from build123d import *

# Parameters (mm, degrees)
SKICA1_R                 = 26
P_IDAT_VYSUNUT_M1_DEPTH  = 90
ZAOBLIT1_R               = 2
SKICA2_R                 = 13
P_IDAT_VYSUNUT_M2_DEPTH  = 6.5
SKICA4_R                 = 1.6
ODEBRAT_VYSUNUT_M1_DEPTH = 10
P_IDAT_START             = 6.5
SKICA5_R                 = 13
P_IDAT_VYSUNUT_M4_DEPTH  = 6.5
ZKOSEN_1_SIZE            = 0.5
SKICA8_R                 = 4
ODEBRAT_VYSUNUT_M3_DEPTH = 110.366356825


with BuildPart() as part:
    # Skica1 → Přidat vysunutím1 (new body)
    with BuildSketch(Plane.XY):
        with Locations(Location((0, 0, 0), (0, 0, 180))):
            Circle(SKICA1_R)
    extrude(amount=P_IDAT_VYSUNUT_M1_DEPTH)

    # Zaoblit1
    zaoblit1_edges = [part.edges().sort_by_distance(p)[0] for p in [
        (26, 0, 0),
        (26, 0, 90),
    ]]
    fillet(zaoblit1_edges, radius=ZAOBLIT1_R)

    # Skica2 → Přidat vysunutím2 (add)
    with BuildSketch(Plane(origin=(0, 0, 0), x_dir=(-1, 0, 0), z_dir=(0, 0, -1))):
        with Locations(Location((0, 0, 0), (0, 0, 180))):
            Circle(SKICA2_R)
    extrude(amount=P_IDAT_VYSUNUT_M2_DEPTH)

    # Skica4 → Odebrat vysunutím1 (cut)
    with BuildSketch(Plane(origin=(0, 0, 0), x_dir=(-1, 0, 0), z_dir=(0, 0, -1))):
        with Locations((-17.5, 0)):
            Circle(SKICA4_R)
        with Locations((0, 17.5)):
            Circle(SKICA4_R)
        with Locations((17.5, 0)):
            Circle(SKICA4_R)
        with Locations((0, -17.5)):
            Circle(SKICA4_R)
    extrude(amount=-ODEBRAT_VYSUNUT_M1_DEPTH, mode=Mode.SUBTRACT)

    # Skica5 → Přidat vysunutím4 (add)
    with BuildSketch(Plane.XY.offset(90).offset(P_IDAT_START)):
        Circle(SKICA5_R)
    extrude(amount=-P_IDAT_VYSUNUT_M4_DEPTH)

    # Zkosení1
    zkosen_1_edges = [part.edges().sort_by_distance(p)[0] for p in [
        (-13, 0, -6.5),
        (-13, 0, 96.5),
    ]]
    chamfer(zkosen_1_edges, length=ZKOSEN_1_SIZE)

    # Skica8 → Odebrat vysunutím3 (cut, through all)
    with BuildSketch(Plane(origin=(0, 0, -6.5), x_dir=(-1, 0, 0), z_dir=(0, 0, -1))):
        Circle(SKICA8_R)
    extrude(amount=-ODEBRAT_VYSUNUT_M3_DEPTH, mode=Mode.SUBTRACT)


solid = part.part
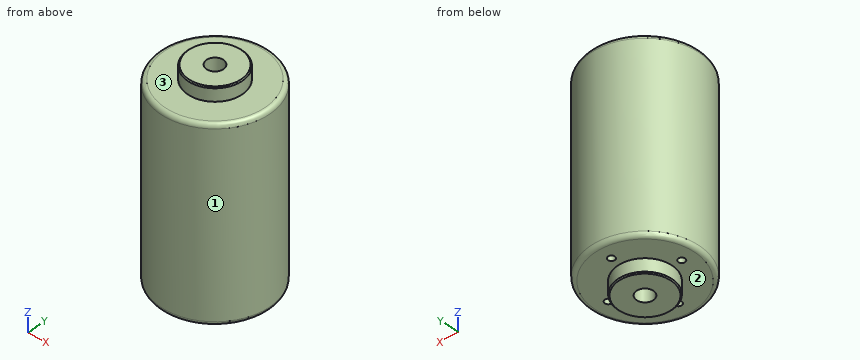
Part model, mm, in its own coordinate system. Face numbers are marked on the shaded views. A direction names the side the tool comes from. Coordinates: 2 decimals unless noted, no trailing zeros. Order: outer loops, then holes, each group sorted by start corner. A loop starts at its lowest first (then second) coordinate and runs counter-clockwise, first axis right, second up.
(1) Pin check, flat tips, straight feed: pin 1 Ø6.5 at (x, y) = (0, 0) entering from +Z; pin 2 Ø1.6 at (x, y) = (0.5, -17.5) entering from -Z; pin 3 Ø2.5 at (x, y) = (18, -0.5) entering from -Z; pin 4 Ø2 at (y, z) = (-13.5, 22) entering from +X. Stop position of each tip, or through.
Check sheet entries:
pin 1: passes through
pin 2: stops at z = 10
pin 3: stops at z = 0
pin 4: stops at x = 22.8
(2) Probe L1, parallel to Y at x = 0, z = 64.5; L2, parallel to Z at x = 20.5, y = 0.5; L3, parallel to Y at x = -3, z = 24. List the from-to ranges inside material, lowest first.
Check sheet entries:
L1: y = -26 to -4, 4 to 26
L2: z = 0 to 90
L3: y = -25.83 to -2.65, 2.65 to 25.83
(3) Slice it at B-B, the plane z = 47. Write the cut outline in (x, y).
Check sheet entries:
outline: circle Ø52 at (0, 0); hole circle Ø8 at (0, 0)
(4) Tool access for the marked faces 1, 2 and 3: list every direction of +Z, -Z, +X, -X, +Y, -Y with a clear straight run to the whole face (end or side of a thin tool).
Check sheet entries:
face 1: +Z, -Z
face 2: -Z
face 3: +Z
